Could you check a few things on this drawing? It's one solid part, dimensions in mm from its lowest x, y, z. A direction names the side the tool comes from. Coordinates: 2 decimals unless noted, no trailing zeros. Order: outer loops, then holes, each group sorted by start corner. A loop starts at its lowest first (then second) coordinate and runs counter-clockwise, first axis right, second up.
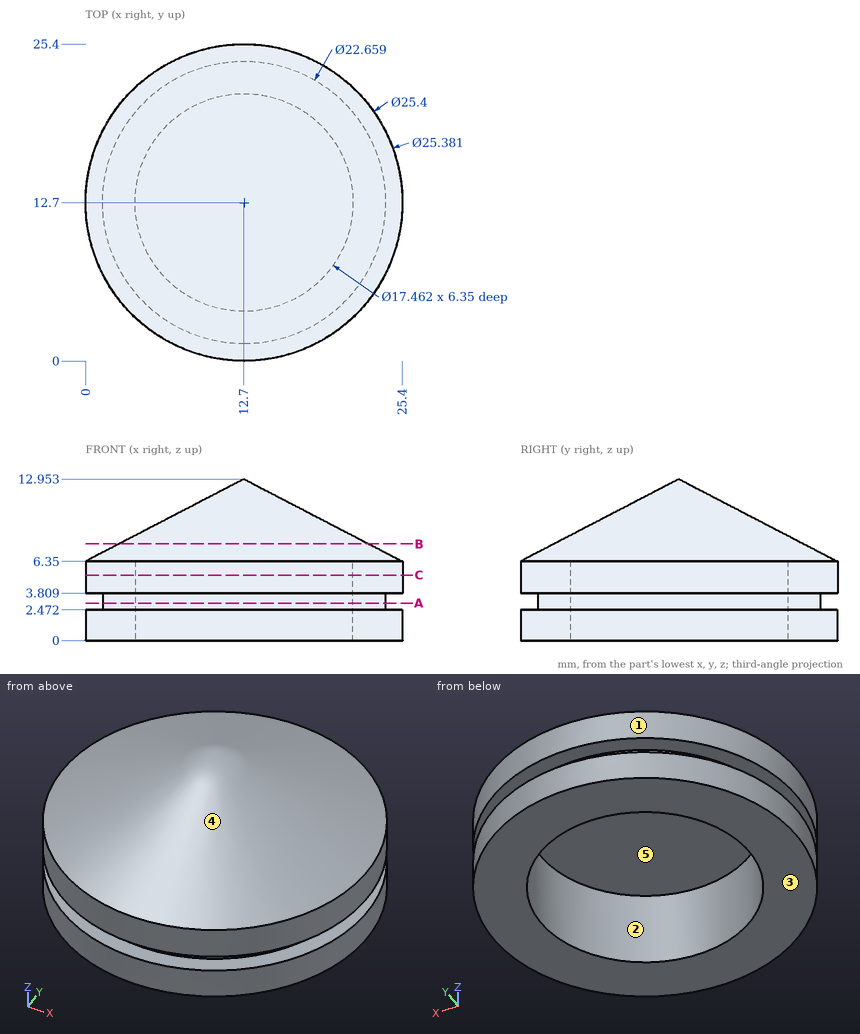
1. Please list where these lines run through material, in increasing order: probe 1 along Y at (x, z) = (17.5, 1) (1 decimal); probe 2 along X at (y, z) = (12.25, 5.5); probe 3 along X at (y, z) = (5.75, 1.25) (1 decimal).
Completed:
probe 1: y = 0.9 to 5.4, 20 to 24.5
probe 2: x = 0.01 to 3.98, 21.42 to 25.39
probe 3: x = 2.1 to 7.4, 18 to 23.3
2. Imagine slicing it at C-C on z = 5.25. Please give me the cut outline in (x, y), then the cut area to 3 significant figures.
Completed:
outline: circle Ø25.4 at (12.7, 12.7); hole circle Ø17.46 at (12.7, 12.7)
area: 267 mm2
3. Imagine slicing it at A-A on z = 3. Please give me the cut outline in (x, y).
Completed:
outline: circle Ø22.66 at (12.7, 12.7); hole circle Ø17.46 at (12.7, 12.7)
4. Thinking about a two-plate mould opening in Y: for the marked faces 1, 2 and 3, which applies, pulls with the +Y half, pulls with the -Y half, needs draft (parallel to the pull), parting line crosses it, or undercut?
Completed:
face 1: parting line crosses it
face 2: undercut
face 3: needs draft
5. Imagine slicing it at B-B on z = 7.75. Please give me the cut outline in (x, y) (1 decimal).
Completed:
outline: circle Ø20 at (12.7, 12.7)
6. I'm going to push flat-ended pins straight in: pin 1 (6 mm diameter, centred on x = 20, y = 18, fed in from +Z); pin 2 (7.5 mm diameter, centred on x = 8.5, y = 16, fed in from +Z) (1 decimal); pin 3 (1 mm diameter, centred on y = 17.5, z = 3.5, fed in from +X); pin 4 (8 mm diameter, centred on x = 14, y = 12, fed in from +Z). Where does each tip first touch, or does it pass through?
Completed:
pin 1: stops at z = 9.82
pin 2: stops at z = 12.1
pin 3: stops at x = 24.61
pin 4: stops at z = 12.95
7. On a 3-axis mill with a long thin cutter (end or side, diameter ignored), from which of +Z, -Z, +X, -X, +Y, -Y can I reach the whole of each face in a straight line? I mean the marked faces 4 and 5. Say none if no direction works.
Completed:
face 4: +Z
face 5: -Z
